from build123d import *

# Parameters (mm, degrees)
F0_W     = 82.026482
F0_H     = 62.353476
F1_DEPTH = 50.8
F2_R     = 12.7


with BuildPart() as f1:
    # F0 (on Top) → F1 (new body)
    with BuildSketch(Plane.XY):
        Rectangle(F0_W, F0_H)
    extrude(amount=F1_DEPTH)

    # F2
    f2_edges = [f1.edges().sort_by_distance(p)[0] for p in [
        (41.013241, 0, 50.8),
        (0, 31.176738, 50.8),
        (-41.013241, 0, 50.8),
        (0, -31.176738, 50.8),
    ]]
    fillet(f2_edges, radius=F2_R)

    # F3: F1 across plane


with BuildPart() as f1_1:
    add(f1.part)
    add(f1.part.mirror(Plane.XY))


solid = f1_1.part
Design review of the part built by this model. Coordinates are the model's own, in mm. Round coordinates to 2 decimals unless told otherwise and drop trailing zeros. Loops run counter-clockwise (first coordinate to the right, second up) from the corner with the lowest first, then second, coordinate; pieces in that order, holes last. Notation, with made-up numbers: (37, 4.5) -> (46, 4.5) arc R5 cw to (46, 13.5) -> close; hole circle Ø4 at (89.5, 68). An arc over 180 degrees is marked (long way). Use one line per item in the form item = value. Start each with the question number.
Q1. Wall thickness on line 1 along X through (y, z) = (-10.5, -46); line 2 along Z through (x, y) = (-30, 14.5); line 3 along X through (y, z) = (-9, 39): over which ranges is each line inside the solid? List them lowest first. Write a range as [from, to].
Q2. We need section A-A on x = 15.5. Give the boundary of the cut face in (y, z).
Q3. We need section B-B on y = -13. Give the boundary of the cut face in (x, z).
Calculated:
q1.line_1 = [-38.26, 38.26]
q1.line_2 = [-50.69, 50.69]
q1.line_3 = [-40.98, 40.98]
q2.outline = (-31.18, -38.1) arc R12.7 ccw to (-18.48, -50.8) -> (18.48, -50.8) arc R12.7 ccw to (31.18, -38.1) -> (31.18, 38.1) arc R12.7 ccw to (18.48, 50.8) -> (-18.48, 50.8) arc R12.7 ccw to (-31.18, 38.1) -> close
q3.outline = (-41.01, -38.1) arc R12.7 ccw to (-28.31, -50.8) -> (28.31, -50.8) arc R12.7 ccw to (41.01, -38.1) -> (41.01, 38.1) arc R12.7 ccw to (28.31, 50.8) -> (-28.31, 50.8) arc R12.7 ccw to (-41.01, 38.1) -> close
